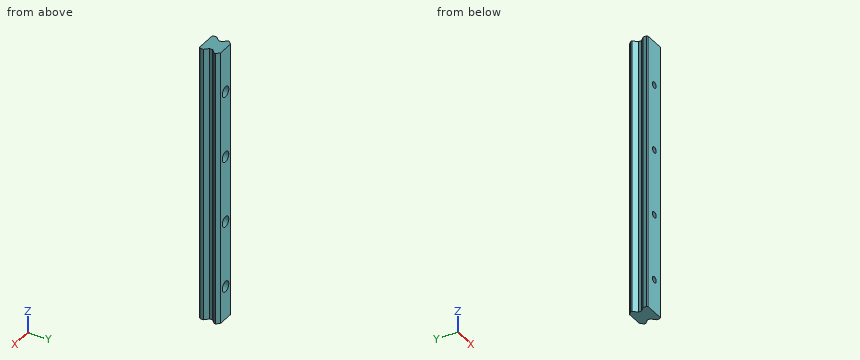
from build123d import *

# Parameters (mm, degrees)
BOSS_EXTRUDE1_DEPTH = 250
LPATTERN2_COUNT     = 4
LPATTERN2_PITCH     = 60


with BuildPart() as part:
    # Sketch1 → Boss-Extrude1 (new body)
    with BuildSketch(Plane.XY):
        Polygon((0, 18), (0, 0), (9, 0), (10.018233765, 1.018233765), (10.018233765, 4.018233765), (6.55, 7.48646753), (6.55, 10.41646753), (10.018233765, 13.884701295), (10.018233765, 15.214701295), (7.16, 18), align=None)
        Polygon((-9, 0), (0, 0), (0, 18), (-7.16, 18), (-10.018233765, 15.214701295), (-10.018233765, 13.884701295), (-6.55, 10.41646753), (-6.55, 7.48646753), (-10.018233765, 4.018233765), (-10.018233765, 1.018233765), align=None)
    extrude(amount=BOSS_EXTRUDE1_DEPTH)

    # Sketch4 → Hole1 (revolve, cut)
    with BuildSketch(Plane(origin=(0, 18, 30), x_dir=(0, 0, 1), z_dir=(1, 0, 0))):
        Polygon((0, 0), (0, 19.652366702), (2.75, 18), (2.75, 8.5), (4.75, 8.5), (4.75, 0), align=None)
    hole1 = revolve(axis=Axis((0, 29.310875039, 30), (0, -1, 0)), mode=Mode.SUBTRACT)

    # LPattern2: Hole1 ×4
    with Locations(*[(0, 0, i * LPATTERN2_PITCH) for i in range(1, LPATTERN2_COUNT)]):
        add(hole1, mode=Mode.SUBTRACT)


solid = part.part
Verification items for the finished model (mm, model axes). Coordinates: 2 decimals unless noted, no trailing zeros. Order: outer loops, then holes, each group sorted by start corner. A loop starts at its lowest first (then second) coordinate and runs counter-clockwise, first axis right, second up. Notation, with made-up numbers: (28.5, 2) -> (64.5, 2) arc R33 ccw to (64.5, 40) -> close; hole circle Ø10 at (-10.75, 4). An arc over 180 degrees is marked (long way). Use CSV: the item, a comma, the result in double quotes. Start each with the question number.
Q1. Section check B-B, the plane z = 191. Record the cut outline in (x, y), and give its area (3 significant figures).
Q2. Thickness scan on line 1 along Z through (x, y) = (0, 16); line 2 along Z through (x, y) = (0, 2.25); line 3 along X through (y, z) = (3, 90). Record the ranges inside material, lowest first.
Q3. Depth check by flat-ended pin: P1, Ø3, axis at x = 1.5, z = 92, coming from the +Y side; P2, Ø1, axis at x = -7.5, z = 162, coming from the +Y side; P3, Ø0.9, axis at y = 9.5, z = 135.5, coming from the -X side; P4, Ø3, axis at y = 9, z = 150, coming from the +X side. Enter the tip coordinate at first touch or a pass-through.
Q4. Section check A-A, the plane z = 90. Record the cut outline in (x, y), and give its area (3 significant figures).
Returned:
1,outline,"(-10.02, 1.02) -> (-9, 0) -> (9, 0) -> (10.02, 1.02) -> (10.02, 4.02) -> (6.55, 7.49) -> (6.55, 10.42) -> (10.02, 13.88) -> (10.02, 15.21) -> (7.16, 18) -> (-7.16, 18) -> (-10.02, 15.21) -> (-10.02, 13.88) -> (-6.55, 10.42) -> (-6.55, 7.49) -> (-10.02, 4.02) -> close"
1,area,"307 mm^2"
2,line 1,"z = 0 to 25.25, 34.75 to 85.25, 94.75 to 145.25, 154.75 to 205.25, 214.75 to 250"
2,line 2,"z = 0 to 27.25, 32.75 to 87.25, 92.75 to 147.25, 152.75 to 207.25, 212.75 to 250"
2,line 3,"x = -10.02 to -2.75, 2.75 to 10.02"
3,P1,"stops at y = 9.5"
3,P2,"stops at y = 18"
3,P3,"stops at x = -6.55"
3,P4,"stops at x = 6.63"
4,outline,"(-10.02, 1.02) -> (-9, 0) -> (-2.75, 0) -> (-2.75, 9.5) -> (-4.75, 9.5) -> (-4.75, 18) -> (-7.16, 18) -> (-10.02, 15.21) -> (-10.02, 13.88) -> (-6.55, 10.42) -> (-6.55, 7.49) -> (-10.02, 4.02) -> close; (2.75, 0) -> (9, 0) -> (10.02, 1.02) -> (10.02, 4.02) -> (6.55, 7.49) -> (6.55, 10.42) -> (10.02, 13.88) -> (10.02, 15.21) -> (7.16, 18) -> (4.75, 18) -> (4.75, 9.5) -> (2.75, 9.5) -> close"
4,area,"174 mm^2"
